```python
from build123d import *

# Parameters (mm, degrees)
SZKIC1_W                    = 100
SZKIC1_H                    = 120
DODANIE_WYCI_GNI_CIE3_DEPTH = 2
SZKIC3_R                    = 5
SZKIC3_R_2                  = 2.5
DODANIE_WYCI_GNI_CIE4_DEPTH = 4
DODANIE_WYCI_GNI_CIE5_DEPTH = 16
SZKIC6_W                    = 94
SZKIC6_H                    = 5
DODANIE_WYCI_GNI_CIE6_DEPTH = 4
SZKIC7_W                    = 112.4
SZKIC7_H                    = 5
DODANIE_WYCI_GNI_CIE7_DEPTH = 3
SZKIC8_W                    = 112.4
SZKIC8_H                    = 5
DODANIE_WYCI_GNI_CIE8_DEPTH = 3
WYTNIJ_WYCI_GNI_CIE1_DEPTH  = 2.5
SZKIC11_W                   = 6
SZKIC11_H                   = 3
SZKIC11_H_2                 = 2.6
WYTNIJ_WYCI_GNI_CIE3_DEPTH  = 1


with BuildPart() as part:
    # Szkic1 → Dodanie-wyciągnięcie3 (new body)
    with BuildSketch(Plane(origin=(0, 0, 0), x_dir=(1, 0, 0), z_dir=(0, 1, 0))):
        with Locations((-26.162790698, -20.11627907)):
            Rectangle(SZKIC1_W, SZKIC1_H)
    extrude(amount=DODANIE_WYCI_GNI_CIE3_DEPTH)

    # Szkic3 → Dodanie-wyciągnięcie4 (add)
    with BuildSketch(Plane(origin=(0, 2, 0), x_dir=(1, 0, 0), z_dir=(0, 1, 0))):
        with Locations((-67.162790698, 28.28372093)):
            Circle(SZKIC3_R)
        with Locations((-67.162790698, 28.28372093)):
            Circle(SZKIC3_R_2, mode=Mode.SUBTRACT)
        with Locations((4.207209302, 28.28372093)):
            Circle(SZKIC3_R)
        with Locations((4.207209302, 28.28372093)):
            Circle(SZKIC3_R_2, mode=Mode.SUBTRACT)
        with Locations((4.207209302, -56.71627907)):
            Circle(SZKIC3_R)
        with Locations((4.207209302, -56.71627907)):
            Circle(SZKIC3_R_2, mode=Mode.SUBTRACT)
        with Locations((-67.162790698, -56.71627907)):
            Circle(SZKIC3_R)
        with Locations((-67.162790698, -56.71627907)):
            Circle(SZKIC3_R_2, mode=Mode.SUBTRACT)
    extrude(amount=DODANIE_WYCI_GNI_CIE4_DEPTH)

    # Szkic4 → Dodanie-wyciągnięcie5 (add)
    with BuildSketch(Plane(origin=(0, 2, 0), x_dir=(1, 0, 0), z_dir=(0, 1, 0))):
        Polygon((-76.162790698, 39.88372093), (-76.162790698, -80.11627907), (-73.162790698, -80.11627907), (-73.162790698, -76.51627907), (-73.162790698, 36.28372093), (20.837209302, 36.28372093), (20.837209302, -76.51627907), (20.837209302, -80.11627907), (23.837209302, -80.11627907), (23.837209302, 39.88372093), align=None)
    extrude(amount=DODANIE_WYCI_GNI_CIE5_DEPTH)

    # Szkic6 → Dodanie-wyciągnięcie6 (add)
    with BuildSketch(Plane.XY.offset(-36.28372093)):
        with Locations((-26.162790698, 15.5)):
            Rectangle(SZKIC6_W, SZKIC6_H)
    extrude(amount=DODANIE_WYCI_GNI_CIE6_DEPTH)

    # Szkic7 → Dodanie-wyciągnięcie7 (add)
    with BuildSketch(Plane.ZY.offset(-20.837209302)):
        with Locations((23.91627907, 15.5)):
            Rectangle(SZKIC7_W, SZKIC7_H)
    extrude(amount=DODANIE_WYCI_GNI_CIE7_DEPTH)

    # Szkic8 → Dodanie-wyciągnięcie8 (add)
    with BuildSketch(Plane(origin=(-73.162790698, 0, 0), x_dir=(0, 0, -1), z_dir=(1, 0, 0))):
        with Locations((-23.91627907, 15.5)):
            Rectangle(SZKIC8_W, SZKIC8_H)
    extrude(amount=DODANIE_WYCI_GNI_CIE8_DEPTH)

    # Szkic10 → Wytnij-wyciągnięcie1 (cut)
    with BuildSketch(Plane(origin=(0, 18, 0), x_dir=(1, 0, 0), z_dir=(0, 1, 0))):
        Polygon((-70.162790698, -80.11627907), (-72.972722391, -80.11627907), (-72.972722391, 35.28372093), (20.837209302, 35.28372093), (20.837209302, -80.11627907), (17.837209302, -80.11627907), (17.837209302, 32.28372093), (-70.162790698, 32.28372093), align=None)
    extrude(amount=-WYTNIJ_WYCI_GNI_CIE1_DEPTH, mode=Mode.SUBTRACT)

    # Szkic11 → Wytnij-wyciągnięcie3 (cut)
    with BuildSketch(Plane(origin=(0, 15.5, 0), x_dir=(1, 0, 0), z_dir=(0, 1, 0))):
        with Locations((-56.010736052, 33.78372093)):
            Rectangle(SZKIC11_W, SZKIC11_H)
        with Locations((-56.010736052, 36.58372093)):
            Rectangle(SZKIC11_W, SZKIC11_H_2)
        with Locations((-36.048749714, 33.78372093)):
            Rectangle(SZKIC11_W, SZKIC11_H)
        with Locations((-36.048749714, 36.58372093)):
            Rectangle(SZKIC11_W, SZKIC11_H_2)
        with Locations((-16.086763375, 33.78372093)):
            Rectangle(SZKIC11_W, SZKIC11_H)
        with Locations((-16.086763375, 36.58372093)):
            Rectangle(SZKIC11_W, SZKIC11_H_2)
        with Locations((3.875222964, 33.78372093)):
            Rectangle(SZKIC11_W, SZKIC11_H)
        with Locations((3.875222964, 36.58372093)):
            Rectangle(SZKIC11_W, SZKIC11_H_2)
    extrude(amount=-WYTNIJ_WYCI_GNI_CIE3_DEPTH, mode=Mode.SUBTRACT)


solid = part.part
```
For this review, take the finished solid that the model builds, in its own axes (mm). A direction names the side the tool comes from. Give positions to 0.01 mm unless a question says otherwise; leave off trailing zeros. Order: outer loops, then holes, each group sorted by start corner. A loop starts at its lowest first (then second) coordinate and runs counter-clockwise, first axis right, second up.
1) Take a section at D-D (x = -7). Give the boundary of the cut face in (y, z).
2) Insertion check: pin 1 (2 mm diameter, centred on x = -20, y = 14, fed in from +Z); pin 2 (8 mm diameter, centred on x = 4, z = -26.5, fed in from +Y); pin 3 (7 mm diameter, centred on x = -66.5, z = 15.5, fed in from +Y). Each pin has a flat end and moves straight along its axis. Give the tip position at first contact, or say it passes through.
3) Take a section at A-A (z = 4.5). Give the boundary of the cut face in (x, y).
4) Take a section at C-C (x = -36). Give the boundary of the cut face in (y, z).
5) The part is to be moulded in two halves that separate along X. For faces 5 (the face through (19, 15.5, 14)), 6 (the face through (-26.4, 1.6, 80.116)), 7 (the face through (-46, 15.5, -34)), say which applies: released by +X, released by -X, zero draft, split by the parting line, or undercut.
6) Wall thickness on line 1 (X direction, y = 3, z = 33.5); line 2 (X direction, y = 15.75, z = 31.5); line 3 (Y direction, x = -25.5, z = -9): over which ranges is each line inside the solid? List them lowest first.
7) For faces 1 (the face through (-70.163, 14, 25)), 2 (the face through (-27, 0, 19)), 3 (the face through (-56, 15.5, -37)), 4 (the face through (5.551, 3.972, -30.392)), list the 3-axis set-ups (+Z, -Z, +X, -X, +Y, -Y) from which the entire face can be reached by the end or side of a thin tool; tool diameter is ignored.
8) Take a section at B-B (y = 11). Give the boundary of the cut face in (x, z), then the cut area to 3 significant figures.
Derived:
1. outline: (0, -39.88) - (18, -39.88) - (18, -35.28) - (15.5, -35.28) - (15.5, -32.28) - (13, -32.28) - (13, -36.28) - (2, -36.28) - (2, 80.12) - (0, 80.12) - close
2. pin 1: stops at z = -32.28
2. pin 2: stops at y = 6
2. pin 3: stops at y = 2
3. outline: (-76.16, 0) - (23.84, 0) - (23.84, 18) - (20.84, 18) - (20.84, 15.5) - (17.84, 15.5) - (17.84, 13) - (20.84, 13) - (20.84, 2) - (-73.16, 2) - (-73.16, 13) - (-70.16, 13) - (-70.16, 15.5) - (-72.97, 15.5) - (-72.97, 18) - (-76.16, 18) - close
4. outline: (0, -39.88) - (18, -39.88) - (18, -35.28) - (15.5, -35.28) - (15.5, -37.88) - (14.5, -37.88) - (14.5, -32.28) - (13, -32.28) - (13, -36.28) - (2, -36.28) - (2, 80.12) - (0, 80.12) - close
5. face 5: undercut
5. face 6: zero draft
5. face 7: undercut
6. line 1: x = -76.16 to -73.16, 20.84 to 23.84
6. line 2: x = -76.16 to -72.97, 20.84 to 23.84
6. line 3: y = 0 to 2
7. face 1: +Z, +Y
7. face 2: +Z, -Z, +X, -X, -Y
7. face 3: +Z
7. face 4: +Y
8. outline: (-76.16, -39.88) - (23.84, -39.88) - (23.84, 80.12) - (20.84, 80.12) - (20.84, -36.28) - (-73.16, -36.28) - (-73.16, 80.12) - (-76.16, 80.12) - close
8. area: 1,060 mm2
